Print and shaded views of the part. All mm, measured from the part's lowest x, y and z. A direction names the side the tool comes from. Round coordinates to 2 decimals unless told otherwise and drop trailing zeros. Order: outer loops, then holes, each group sorted by start corner. A loop starts at its lowest first (then second) coordinate and runs counter-clockwise, first axis right, second up. Notation, with made-up numbers: (19.25, 8.5) - (61.25, 8.5) arc R17 cw to (61.25, 19.5) - close; hole circle Ø8 at (41, 72). An arc over 180 degrees is marked (long way). Write item = value, one per line.
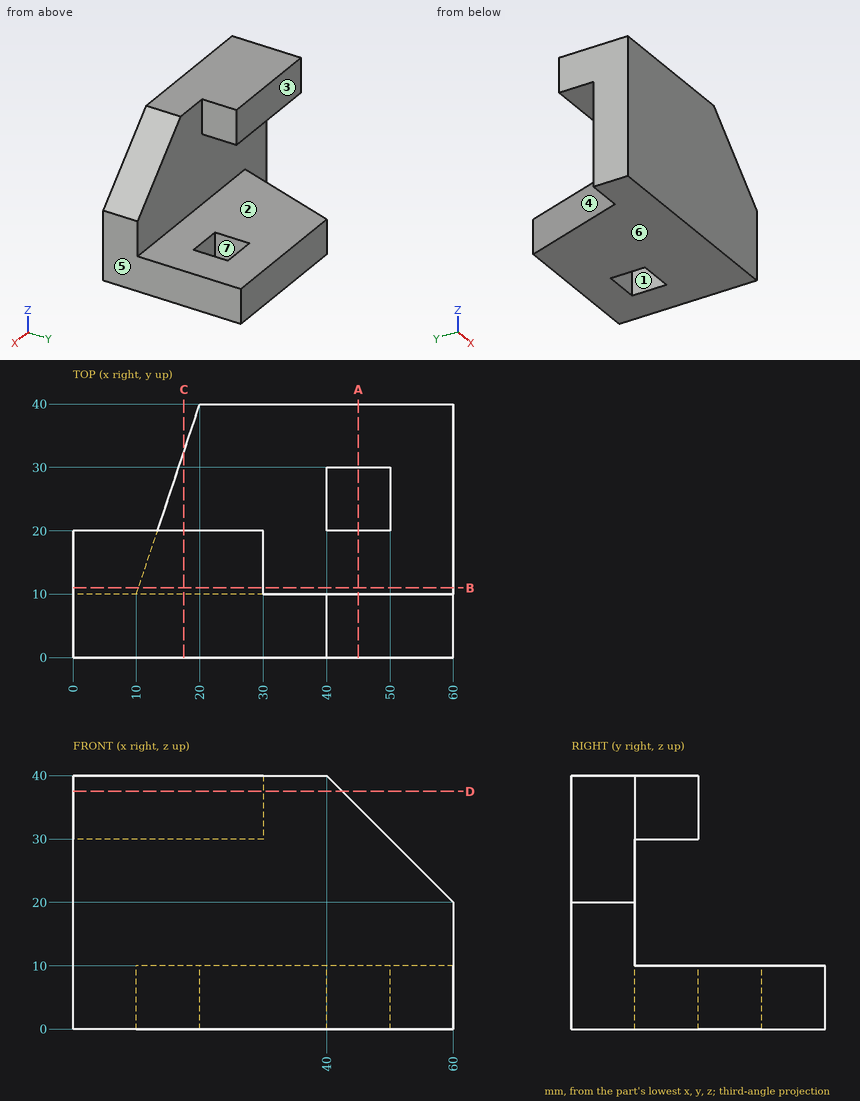
(1) Band-saw the part on B-B on y = 11. List the corners of the cut face in (x, z), plus the area to 3 significant figures.
Solved:
outline = (0, 30) - (30, 30) - (30, 40) - (0, 40) - close; (10.33, 0) - (60, 0) - (60, 10) - (10.33, 10) - close
area = 797 mm²
(2) Probe line 1 along Z through (x, y) = (58.5, 17.5); line 2 along X through (y, z) = (14.5, 31). List the from-to ranges inside material, lowest first.
Solved:
line_1 = 0 to 10
line_2 = 0 to 30
(3) Band-saw the part on A-A on x = 45. List the corners of the cut face in (y, z), plus the area to 3 significant figures.
Solved:
outline = (0, 0) - (20, 0) - (20, 10) - (10, 10) - (10, 35) - (0, 35) - close; (30, 0) - (40, 0) - (40, 10) - (30, 10) - close
area = 550 mm²
(4) Pull direction X, two halves, no side cores. Call the marked faces 5, 6 and 7: released by +X, released by -X, zero draft, split by the parting line, or undercut.
Solved:
face_5 = released by +X
face_6 = zero draft
face_7 = undercut
(5) Drop flat-ended pins along their axis: pin 1 (8 mm diameter, centred on y = 25, z = 4.5, fed in from -X); pin 2 (11 mm diameter, centred on x = 17, z = 32.5, fed in from +Y); pin 3 (5 mm diameter, centred on x = 49.5, y = 6, fed in from -Z); pin 4 (5 mm diameter, centred on x = 21.5, z = 24.5, fed in from +Y). Give the stop position or say it passes through.
Solved:
pin_1 = 13.67
pin_2 = 20
pin_3 = 0
pin_4 = 10
(6) Tool access for the marked faces 1, 2, 3 and 4: list every direction of +Z, -Z, +X, -X, +Y, -Y with a clear straight run to the whole face (end or side of a thin tool).
Solved:
face_1 = +Z, -Z
face_2 = +X, -X, +Y
face_3 = +Z, +X, -X, +Y
face_4 = -Z, -X, +Y
(7) Band-saw the part on D-D on z = 37.5. List the corners of the cut face in (x, y), plus the area to 3 significant figures.
Solved:
outline = (0, 0) - (42.5, 0) - (42.5, 10) - (30, 10) - (30, 20) - (0, 20) - close
area = 725 mm²
(8) Band-saw the part on C-C on x = 17.5. List the corners of the cut face in (y, z), plus the area to 3 significant figures.
Solved:
outline = (0, 0) - (32.5, 0) - (32.5, 10) - (10, 10) - (10, 30) - (20, 30) - (20, 40) - (0, 40) - close
area = 725 mm²
